```python
from build123d import *

# Parameters (mm, degrees)
SKETCH1_R           = 14.2875
BOSS_EXTRUDE1_DEPTH = 7.239
SKETCH2_R           = 1.5875
CUT_EXTRUDE1_DEPTH  = 25.857147795


with BuildPart() as part:
    # Sketch1 → Boss-Extrude1 (new, symmetric)
    with BuildSketch(Plane.XY):
        Circle(SKETCH1_R)
    extrude(amount=BOSS_EXTRUDE1_DEPTH, both=True)

    # Sketch2 → Cut-Extrude1 (cut, through all)
    with BuildSketch(Plane.XY.offset(7.239)):
        with Locations((-10.31875, 0)):
            Circle(SKETCH2_R)
        with Locations((-5.159375, 8.936299635)):
            Circle(SKETCH2_R)
        with Locations((5.159375, 8.936299635)):
            Circle(SKETCH2_R)
        with Locations((10.31875, 0)):
            Circle(SKETCH2_R)
        with Locations((5.159375, -8.936299635)):
            Circle(SKETCH2_R)
        with Locations((-5.159375, -8.936299635)):
            Circle(SKETCH2_R)
        Polygon((0, 7.332348419), (-6.35, 3.666174209), (-6.35, -3.666174209), (0, -7.332348419), (6.35, -3.666174209), (6.35, 3.666174209), align=None)
    extrude(amount=-CUT_EXTRUDE1_DEPTH, mode=Mode.SUBTRACT)


solid = part.part
```
Model file for the job. Use its own axes, mm. A direction names the side the tool comes from. Round coordinates to 2 decimals unless told otherwise and drop trailing zeros. Write each loop counter-clockwise with the first axis right and the second up, starting at its lowest first coordinate (ties: lowest second). Pieces come first, ordered by that corner, then holes. Notation, with made-up numbers: M -15.5,68 L 12.5,68 A19 cw 12.5,86 Z; hole C 37.25,-11 d1. An arc over 180 degrees is marked long. Put each result on its own line as item: value.
Item 1: Cut at A-A (y = 0). List the corners of the cut face in (x, z), and give its area (3 significant figures).
Responses:
outline: M -14.29,-7.24 L -11.91,-7.24 L -11.91,7.24 L -14.29,7.24 Z; M -8.73,-7.24 L -6.35,-7.24 L -6.35,7.24 L -8.73,7.24 Z; M 6.35,-7.24 L 8.73,-7.24 L 8.73,7.24 L 6.35,7.24 Z; M 11.91,-7.24 L 14.29,-7.24 L 14.29,7.24 L 11.91,7.24 Z
area: 138 mm²
Item 2: Cut at C-C (z = -6.5). State how many separate pieces and enclosed holes the cut face has, and give its area (3 significant figures).
Responses:
separate pieces: 1
enclosed holes: 7
area: 454 mm²
Item 3: Cut at D-D (y = -9.75). List the corners of the cut face in (x, z).
Responses:
outline: M -10.44,-7.24 L -6.52,-7.24 L -6.52,7.24 L -10.44,7.24 Z; M -3.8,-7.24 L 3.8,-7.24 L 3.8,7.24 L -3.8,7.24 Z; M 6.52,-7.24 L 10.44,-7.24 L 10.44,7.24 L 6.52,7.24 Z
Item 4: Probe L1, parallel to Y at x = 4.5, z = 2; L2, parallel to Y at x = -5.75, z = -4.5; L3, parallel to X at y = 9.25, z = -3.75. List the from-to ranges inside material, lowest first. Write a range as from..to.
Responses:
L1: -13.56..-10.38, -7.49..-4.73, 4.73..7.49, 10.38..13.56
L2: -13.08..-10.41, -7.46..-4.01, 4.01..7.46, 10.41..13.08
L3: -10.89..-6.72, -3.6..3.6, 6.72..10.89
Item 5: Flat gauge pins, fed straight in: P1, Ø3, axis at y = -6, z = 1.5, coming from the -X side; P2, Ø3, axis at y = -10.5, z = 2, coming from the +X side; P3, Ø4, axis at x = -3, z = 3.5, coming from the +Y side. Where does each tip first touch, or does it go through?
Responses:
P1: x = -13.56
P2: x = 11.1
P3: y = 14.25
Item 6: Tool access for faces 1 (the flat face through (6.35, 0, 0)), 2 (the flat face through (-7, 0, -7.239)): list every direction of +Z, -Z, +X, -X, +Y, -Y with a clear straight run to the whole face (end or side of a thin tool).
Responses:
face 1: +Z, -Z
face 2: -Z, +X, -X, +Y, -Y
Item 7: Cut at B-B (x = 1.75). List the corners of the cut face in (y, z), and give its area (3 significant figures).
Responses:
outline: M -14.18,-7.24 L -6.32,-7.24 L -6.32,7.24 L -14.18,7.24 Z; M 6.32,-7.24 L 14.18,-7.24 L 14.18,7.24 L 6.32,7.24 Z
area: 228 mm²
Item 8: Mould opens along Y. For faces 3 (the flat face through (-7, 0, 7.239)), 4 (the cylindrical face through (-14.274, 0.628, 0.101)), 5 (the flat face through (-3.131, 5.525, 0.101)) say: +Y half, -Y half, draft (parallel to the pull), parting line (faces both ways), or undercut.
Responses:
face 3: draft
face 4: parting line
face 5: undercut
